```python
from build123d import *

# Parameters (mm, degrees)
SKETCH1_W           = 266.7
SKETCH1_H           = 130.0068901
BOSS_EXTRUDE1_DEPTH = 316.09292636
SKETCH2_R           = 4.7625
SKETCH2_R_2         = 12.8984375
CUT_EXTRUDE1_DEPTH  = 266.7
SKETCH3_R           = 12.8984375
SKETCH3_R_2         = 7.3421875
SKETCH3_W           = 78.287500016
SKETCH3_H           = 5.262500016
CUT_EXTRUDE2_DEPTH  = 332.74
SKETCH4_W           = 267.993719028
SKETCH4_H           = 38.1
CUT_EXTRUDE3_DEPTH  = 18.000000068


with BuildPart() as part:
    # Sketch1 → Boss-Extrude1 (new body)
    with BuildSketch(Plane(origin=(0, 0, 0), x_dir=(0, 0, -1), z_dir=(1, 0, 0))):
        Rectangle(SKETCH1_W, SKETCH1_H)
    extrude(amount=BOSS_EXTRUDE1_DEPTH)

    # Sketch2 → Cut-Extrude1 (cut)
    with BuildSketch(Plane.XY.offset(133.35)):
        with Locations((93.639440102, 39.990297972)):
            Circle(SKETCH2_R)
        with Locations((222.453486258, 39.990297972)):
            Circle(SKETCH2_R)
        with Locations((303.39292636, -52.30344505)):
            Circle(SKETCH2_R)
        with Locations((12.7, -52.30344505)):
            Circle(SKETCH2_R)
        with Locations((158.04646318, 35.218991284)):
            Circle(SKETCH2_R_2)
    extrude(amount=-CUT_EXTRUDE1_DEPTH, mode=Mode.SUBTRACT)

    # Sketch3 → Cut-Extrude2 (cut)
    with BuildSketch(Plane(origin=(316.09292636, 0, 0), x_dir=(0, 0, -1), z_dir=(1, 0, 0))):
        with Locations((-114.617463678, 7.67564505)):
            Circle(SKETCH3_R)
        with Locations((37.782536322, 7.67564505)):
            Circle(SKETCH3_R_2)
        with Locations((-38.4175, 7.67564505)):
            Rectangle(SKETCH3_W, SKETCH3_H)
    extrude(amount=-CUT_EXTRUDE2_DEPTH, mode=Mode.SUBTRACT)

    # Sketch4 → Cut-Extrude3 (cut)
    with BuildSketch(Plane.XY.offset(133.35)):
        with Locations((158.04646318, -45.95344505)):
            Rectangle(SKETCH4_W, SKETCH4_H)
    cut_extrude3 = extrude(amount=-CUT_EXTRUDE3_DEPTH, mode=Mode.SUBTRACT)

    # Mirror1: Cut-Extrude3 across plane
    add(cut_extrude3.mirror(Plane.XY), mode=Mode.SUBTRACT)


solid = part.part
```
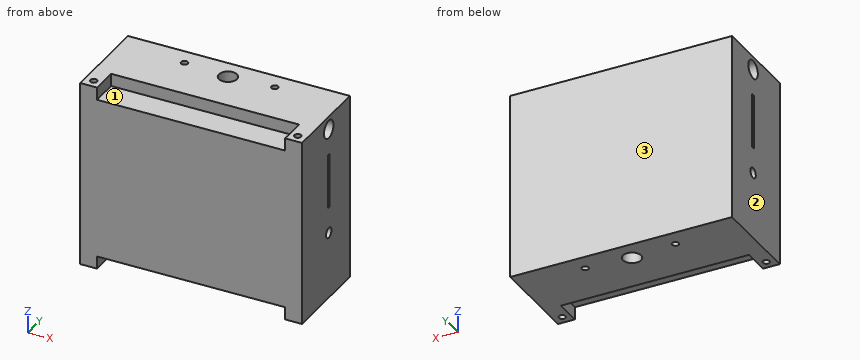
Check sheet for the modelled part. Datum: model origin and axes. Units: mm. Face numbers are marked on the shaded views. Coordinates: 2 decimals unless noted, no trailing zeros. Loops run counter-clockwise (first coordinate to the right, second up) from the corner with the lowest first, then second, coordinate; pieces in that order, holes last. Notation, with made-up numbers: M -4,-7 L 46,-7 A20 cw 46,30 Z; hole C -19,21 d1. An arc over 180 degrees is marked long. Answer as a JSON object with one key per item and string values.
1. Sectioned sample at C-C on y = 31. Record the cut outline in (x, z), and give its area (3 significant figures).
Outcome:
{"outline": "M 0,-133.35 L 145.86,-133.35 L 145.86,133.35 L 0,133.35 Z; M 170.24,-133.35 L 316.09,-133.35 L 316.09,133.35 L 170.24,133.35 Z", "area": "77,800 mm²"}
2. Sectioned sample at A-A on z = 4. Record the cut outline in (x, y) (1 decimal), and give its area (3 significant figures).
Outcome:
{"outline": "M 0,-65 L 316.1,-65 L 316.1,5 L 0,5 Z; M 0,10.3 L 316.1,10.3 L 316.1,65 L 0,65 Z; hole C 12.7,-52.3 d9.5; hole C 93.6,40 d9.5; hole C 158,35.2 d25.8; hole C 222.5,40 d9.5; hole C 303.4,-52.3 d9.5", "area": "38,600 mm²"}
3. Release check for a two-part mould opening along X. For the marked faces 1, 2 and 3 record: pulls with the +X half, pulls with the -X half, needs draft (parallel to the pull), parting line crosses it, or undercut.
Outcome:
{"face 1": "undercut", "face 2": "pulls with the -X half", "face 3": "needs draft"}
4. Scan lines: L1, parallel to Z at x = 242.5, y = 6.5; L2, parallel to Y at x = 287.5, z = 64; L3, parallel to Y at x = 14.5, z = 38. Record each from-to range of solid material in increasing order. Write a range as from..to.
Outcome:
{"L1": "-133.35..-45.03, -30.54..-0.73, 77.56..101.77, 127.46..133.35", "L2": "-65..5.04, 10.31..65", "L3": "-65..-56.71, -47.89..5.04, 10.31..65"}
5. Sectioned sample at B-B on x = 12.7. Record the cut outline in (y, z), and give its area (3 significant figures).
Outcome:
{"outline": "M -65,-133.35 L -57.07,-133.35 L -57.07,133.35 L -65,133.35 Z; M -47.54,-133.35 L 65,-133.35 L 65,133.35 L -47.54,133.35 Z; hole C 7.68,114.62 d25.8; hole C 7.68,-37.78 d14.68; hole M 5.04,-0.73 L 10.31,-0.73 L 10.31,77.56 L 5.04,77.56 Z", "area": "31,000 mm²"}
6. Sectioned sample at D-D on x = 64. Record the cut outline in (y, z).
Outcome:
{"outline": "M -65,-115.35 L -26.9,-115.35 L -26.9,-133.35 L 65,-133.35 L 65,133.35 L -26.9,133.35 L -26.9,115.35 L -65,115.35 Z; hole C 7.68,114.62 d25.8; hole C 7.68,-37.78 d14.68; hole M 5.04,-0.73 L 10.31,-0.73 L 10.31,77.56 L 5.04,77.56 Z"}
7. Depth check by flat-ended pin: P1, Ø20, axis at x = 115, z = 128.5, coming from the -Y side; P2, Ø1, axis at x = 81, y = -34, coming from the +Z side. Enter the tip coordinate at first touch or a pass-through.
Outcome:
{"P1": "y = -26.9", "P2": "z = 115.35"}
